Design review of the part built by this model. Coordinates are the model's own, in mm. A direction names the side the tool comes from. Round coordinates to 2 decimals unless told otherwise and drop trailing zeros. Write each loop counter-clockwise with the first axis right and the second up, starting at its lowest first coordinate (ties: lowest second). Pieces come first, ordered by that corner, then holes. Notation, with made-up numbers: M 49,74.25 L 66,74.25 A18 cw 66,92.25 Z; hole C 32,30.5 d5. An arc over 180 degrees is marked long. Use CSV: the item, a comma, the result in double quotes.
from build123d import *

# Parameters (mm, degrees)
SKETCH_1_R               = 6
EXTRUDE_1_DEPTH          = 5
CUT_EXTRUDE_1_DEPTH      = 142.435598161
CUT_EXTRUDE_1_DEPTH_BACK = 142.435598161
SKETCH_5_W               = 5
SKETCH_5_H               = 50
SKETCH_6_R               = 111.64768953
EXTRUDE_4_DEPTH          = 5
F_3_0MM_1_D              = 3
PATTERN_CIRCULAR_1_COUNT = 3
HOLE_WIZARD_M4_1_D       = 3.3


with BuildPart() as part:
    # 草圖1 → 填料-伸長1 (new body)
    with BuildSketch(Plane(origin=(0, 0, 0), x_dir=(1, 0, 0), z_dir=(0, 1, 0))):
        with BuildLine():
            ThreePointArc((-54.140127389, 84.076433121), (-86.602540378, 50), (-99.882390637, 4.848509122))
            ThreePointArc((-99.882390637, 4.848509122), (-94.722486108, -4.890404948), (-83.701905284, -5.024047358))
            ThreePointArc((-83.701905284, -5.024047358), (-32.475952642, -18.75), (-46.201905284, -69.975952642))
            ThreePointArc((-46.201905284, -69.975952642), (-51.596457973, -79.586876805), (-45.742263248, -88.924942243))
            ThreePointArc((-45.742263248, -88.924942243), (0, -100), (45.742263248, -88.924942243))
            ThreePointArc((45.742263248, -88.924942243), (51.596457973, -79.586876805), (46.201905284, -69.975952642))
            ThreePointArc((46.201905284, -69.975952642), (32.475952642, -18.75), (83.701905284, -5.024047358))
            ThreePointArc((83.701905284, -5.024047358), (94.722486108, -4.890404948), (99.882390637, 4.848509122))
            ThreePointArc((99.882390637, 4.848509122), (86.602540378, 50), (54.140127389, 84.076433121))
            ThreePointArc((54.140127389, 84.076433121), (43.126028135, 84.477281753), (37.5, 75))
            ThreePointArc((37.5, 75), (0, 37.5), (-37.5, 75))
            ThreePointArc((-37.5, 75), (-43.126028135, 84.477281753), (-54.140127389, 84.076433121))
        make_face()
        with Locations(Location((0, 0, 0), (0, 0, 270))):
            Circle(SKETCH_1_R, mode=Mode.SUBTRACT)
    extrude(amount=-EXTRUDE_1_DEPTH)

    # 草圖5 → 除料-伸長1 (cut, two sides: drawn at the far end of the back side and taken through both)
    with BuildSketch(Plane(origin=(0, 0, 0), x_dir=(1, 0, 0), z_dir=(0, 1, 0)).offset(-CUT_EXTRUDE_1_DEPTH_BACK)):
        with BuildLine():
            ThreePointArc((18.659757868, -98.243643236), (-14.320442433, -98.969313065), (-45.742263248, -88.924942243))
            ThreePointArc((-45.742263248, -88.924942243), (-51.596457973, -79.586876805), (-46.201905284, -69.975952642))
            ThreePointArc((-46.201905284, -69.975952642), (-35.201155023, -60.328553588), (-28.729686798, -47.205714191))
            ThreePointArc((-28.729686798, -47.205714191), (-19.144613028, -85.825688538), (18.659757868, -98.243643236))
        make_face()
        with BuildLine():
            ThreePointArc((75.751611869, 65.28164596), (92.870160526, 37.082789592), (99.882390637, 4.848509122))
            ThreePointArc((99.882390637, 4.848509122), (94.722486108, -4.890404948), (83.701905284, -5.024047358))
            ThreePointArc((83.701905284, -5.024047358), (69.846637492, -0.320817698), (55.246191092, -1.277781514))
            ThreePointArc((55.246191092, -1.277781514), (83.899533086, 26.333123041), (75.751611869, 65.28164596))
        make_face()
        Polygon((-20.400635095, 14.665063509), (-22.900635095, 10.334936491), (-66.201905284, 35.334936491), (-63.701905284, 39.665063509), align=None)
        with Locations((0, -50)):
            Rectangle(SKETCH_5_W, SKETCH_5_H)
        Polygon((22.900635095, 10.334936491), (20.400635095, 14.665063509), (63.701905284, 39.665063509), (66.201905284, 35.334936491), align=None)
        with BuildLine():
            ThreePointArc((-37.5, 75), (-34.645482469, 60.649371286), (-26.516504294, 48.483495706))
            ThreePointArc((-26.516504294, 48.483495706), (-64.754920057, 59.492565497), (-94.411369737, 32.961997276))
            ThreePointArc((-94.411369737, 32.961997276), (-78.549718093, 61.886523473), (-54.140127389, 84.076433121))
            ThreePointArc((-54.140127389, 84.076433121), (-43.126028135, 84.477281753), (-37.5, 75))
        make_face()
    extrude(amount=CUT_EXTRUDE_1_DEPTH + CUT_EXTRUDE_1_DEPTH_BACK, mode=Mode.SUBTRACT)

    # 草圖6 → 填料-伸長4 (add)
    # profile 1 of 2: a face of its own
    with BuildSketch(Plane(origin=(0, 0, 0), x_dir=(1, 0, 0), z_dir=(0, 1, 0))):
        with Locations(Location((0, 0, 0), (0, 0, 270))):
            Circle(SKETCH_6_R)
        with BuildLine():
            Line((-64.951905284, -37.5), (-28.729686798, -47.205714191))
            ThreePointArc((-28.729686798, -47.205714191), (-19.144613028, -85.825688538), (18.659757868, -98.243643236))
            ThreePointArc((18.659757868, -98.243643236), (32.536358555, -94.558898957), (45.742263248, -88.924942243))
            ThreePointArc((45.742263248, -88.924942243), (51.596457973, -79.586876805), (46.201905284, -69.975952642))
            ThreePointArc((46.201905284, -69.975952642), (27.772722982, -32.605267792), (55.246191092, -1.277781514))
            ThreePointArc((55.246191092, -1.277781514), (83.899533086, 26.333123041), (75.751611869, 65.28164596))
            ThreePointArc((75.751611869, 65.28164596), (65.622229374, 75.456762534), (54.140127389, 84.076433121))
            ThreePointArc((54.140127389, 84.076433121), (43.126028135, 84.477281753), (37.5, 75))
            ThreePointArc((37.5, 75), (14.350628714, 40.354517531), (-26.516504294, 48.483495706))
            ThreePointArc((-26.516504294, 48.483495706), (-64.754920057, 59.492565497), (-94.411369737, 32.961997276))
            ThreePointArc((-94.411369737, 32.961997276), (-98.158587928, 19.102136424), (-99.882390637, 4.848509122))
            ThreePointArc((-99.882390637, 4.848509122), (-94.722486108, -4.890404948), (-83.701905284, -5.024047358))
            Line((-83.701905284, -5.024047358), (-64.951905284, -37.5))
        make_face(mode=Mode.SUBTRACT)
    # profile 2 of 2: a face of its own
    with BuildSketch(Plane(origin=(0, 0, 0), x_dir=(1, 0, 0), z_dir=(0, 1, 0))):
        with BuildLine():
            Line((-83.701905284, -5.024047358), (-64.951905284, -37.5))
            Line((-64.951905284, -37.5), (-28.729686798, -47.205714191))
            ThreePointArc((-28.729686798, -47.205714191), (-42.123351696, -7.749249739), (-83.701905284, -5.024047358))
        make_face()
    extrude(amount=-EXTRUDE_4_DEPTH)

    # Ø3.0mm 定位孔1 (through all)
    with Locations(Plane(origin=(0, 0, 0), x_dir=(1, 0, 0), z_dir=(0, 1, 0))):
        with Locations((-43.948722523, -67.039547699), (-57.342387421, -27.583083246), (-98.920941009, -24.857880865)):
            f_3_0mm_1 = Hole(F_3_0MM_1_D / 2)

    # 環狀複製排列1: Ø3.0mm 定位孔1 ×3 about axis
    pattern_circular_1_axis = Axis((0, 0, 0), (0, 1, 0))
    for i in range(1, PATTERN_CIRCULAR_1_COUNT):
        add(f_3_0mm_1.rotate(pattern_circular_1_axis, i * 360 / PATTERN_CIRCULAR_1_COUNT), mode=Mode.SUBTRACT)

    # M4 螺紋孔1 (through all)
    with Locations(Plane(origin=(0, 0, 0), x_dir=(1, 0, 0), z_dir=(0, 1, 0))):
        with Locations((0, 12), (12, 0), (0, -12), (-12, 0)):
            Hole(HOLE_WIZARD_M4_1_D / 2)


solid = part.part
1) For pin 1 Ø1.8 at (x, z) = (70.99, 73.24) entering from +Y; pin 2 Ø2 at (x, y) = (-42, -1.5) entering from +Z; pin 3 Ø1.5 at (y, z) = (-1.5, 47.5) entering from +X, all flat-tipped, find the tip position at first contact; note any pin that passes through.
Answers:
pin 1,"through"
pin 2,"z = 103.85"
pin 3,"x = 101.39"
2) Add section B-B on y = -2.9. Give the number of separate pieces and of enclosed holes in the cut face, then the cut area to 3 significant figures.
Answers:
separate pieces,"1"
enclosed holes,"17"
area,"38,200 mm²"
3) Wall thickness on line 1 along Z through (x, y) = (-57, -1.4); line 2 along Z through (x, y) = (-58.5, -0.3); line 3 along X through (y, z) = (-1.1, -12): over which ranges is each line inside the solid? List them lowest first. Write a range as [from, to].
Answers:
line 1,"[-96, -35.8], [-30.02, 26.12], [29.04, 96]"
line 2,"[-95.09, -36.66], [-30.89, 26.63], [28.54, 95.09]"
line 3,"[-111, -25.78], [-21.94, -1.65], [1.65, 21.94], [25.78, 111]"
4) Add section C-C on x = 86. Write out the cut boundary in (y, z).
Answers:
outline,"M -5,-71.2 L 0,-71.2 L 0,71.2 L -5,71.2 Z"
5) Machinability: for faces 4 (the face through (2.5, -3, 50)), 5 (the face through (-23, 0, -2)), which of the approach directions +Z, -Z, +X, -X, +Y, -Y give a long, thin tool a straight path to every point of the face, cutting with its end or side? Answer none if there is none.
Answers:
face 4,"+Y, -Y"
face 5,"+Z, -Z, +X, -X, +Y"
6) Add section A-A on x = 58.5. Write out the cut boundary in (y, z), then the cut area to 3 significant figures.
Answers:
outline,"M -5,-95.09 L 0,-95.09 L 0,-36.66 L -5,-36.66 Z; M -5,-30.89 L 0,-30.89 L 0,95.09 L -5,95.09 Z"
area,"922 mm²"
7) The part is to be moulded in two halves that separate along X. For faces 1 (the face through (4.91, -2.46, -111.54)), 2 (the face through (-23, -5, -2)), 3 (the face through (0, -3, 75)), say which applies: released by +X, released by -X, zero draft, split by the parting line, or undercut.
Answers:
face 1,"split by the parting line"
face 2,"zero draft"
face 3,"undercut"
